from build123d import *

# Parameters (mm, degrees)
F0_R     = 5.0038
F0_R_2   = 5.1038
F0_R_3   = 5.2038
F0_R_4   = 5.3038
F0_R_5   = 5.4038
F0_R_6   = 5.9038
F0_R_7   = 5.8038
F0_R_8   = 5.7038
F0_R_9   = 5.6038
F0_R_10  = 5.5038
F1_DEPTH = 2.9464
F2_R     = 5.9038
F2_R_2   = 5.8038
F2_R_3   = 5.7038
F2_R_4   = 5.6038
F2_R_5   = 5.5038
F2_R_6   = 5.0038
F2_R_7   = 5.1038
F2_R_8   = 5.2038
F2_R_9   = 5.3038
F2_R_10  = 5.4038
F3_DEPTH = 2.54


with BuildPart() as f1:
    # F0 (on Top) → F1 (new body)
    with BuildSketch(Plane.XY):
        with BuildLine():
            Line((27.8450359044, 20.32), (-38.1949640956, 20.32))
            Line((-38.1949640956, 20.32), (-38.1949640956, -1.27))
            ThreePointArc((-38.1949640956, -1.27), (-36.3350921561, -5.7601280605), (-31.8449640956, -7.62))
            Line((-31.8449640956, -7.62), (27.8450359044, -7.62))
            Line((27.8450359044, -7.62), (27.8450359044, 20.32))
        make_face()
        with Locations((-30.5749640956, 0)):
            Circle(F0_R, mode=Mode.SUBTRACT)
        with Locations((-17.8749640956, 0)):
            Circle(F0_R_2, mode=Mode.SUBTRACT)
        with Locations((-5.1749640956, 0)):
            Circle(F0_R_3, mode=Mode.SUBTRACT)
        with Locations((7.5250359044, 0)):
            Circle(F0_R_4, mode=Mode.SUBTRACT)
        with Locations((20.2250359044, 0)):
            Circle(F0_R_5, mode=Mode.SUBTRACT)
        with Locations((-30.5749640956, 12.7)):
            Circle(F0_R_6, mode=Mode.SUBTRACT)
        with Locations((-17.8749640956, 12.7)):
            Circle(F0_R_7, mode=Mode.SUBTRACT)
        with Locations((-5.1749640956, 12.7)):
            Circle(F0_R_8, mode=Mode.SUBTRACT)
        with Locations((7.5250359044, 12.7)):
            Circle(F0_R_9, mode=Mode.SUBTRACT)
        with Locations((20.2250359044, 12.7)):
            Circle(F0_R_10, mode=Mode.SUBTRACT)
    extrude(amount=F1_DEPTH)

    # F2 (on face) → F3 (join)
    with BuildSketch(Plane(origin=(0, 0, 0), x_dir=(1, 0, 0), z_dir=(0, 0, -1))):
        with BuildLine():
            Line((-38.1949640956, 1.27), (-38.1949640956, -20.32))
            Line((-38.1949640956, -20.32), (27.8450359044, -20.32))
            Line((27.8450359044, -20.32), (27.8450359044, 7.62))
            Line((27.8450359044, 7.62), (-31.8449640956, 7.62))
            ThreePointArc((-31.8449640956, 7.62), (-36.3350921561, 5.7601280605), (-38.1949640956, 1.27))
        make_face()
        with Locations((-30.5749640956, -12.7)):
            Circle(F2_R, mode=Mode.SUBTRACT)
        with Locations((-17.8749640956, -12.7)):
            Circle(F2_R_2, mode=Mode.SUBTRACT)
        with Locations((-5.1749640956, -12.7)):
            Circle(F2_R_3, mode=Mode.SUBTRACT)
        with Locations((7.5250359044, -12.7)):
            Circle(F2_R_4, mode=Mode.SUBTRACT)
        with Locations((20.2250359044, -12.7)):
            Circle(F2_R_5, mode=Mode.SUBTRACT)
        with Locations((-30.5749640956, 0)):
            Circle(F2_R_6, mode=Mode.SUBTRACT)
        with Locations((-17.8749640956, 0)):
            Circle(F2_R_7, mode=Mode.SUBTRACT)
        with Locations((-5.1749640956, 0)):
            Circle(F2_R_8, mode=Mode.SUBTRACT)
        with Locations((7.5250359044, 0)):
            Circle(F2_R_9, mode=Mode.SUBTRACT)
        with Locations((20.2250359044, 0)):
            Circle(F2_R_10, mode=Mode.SUBTRACT)
        with Locations((-30.5749640956, 0)):
            Circle(F2_R_6)
        with Locations((-30.5749640956, -12.7)):
            Circle(F2_R)
        with Locations((-17.8749640956, -12.7)):
            Circle(F2_R_2)
        with Locations((-17.8749640956, 0)):
            Circle(F2_R_7)
        with Locations((-5.1749640956, 0)):
            Circle(F2_R_8)
        with Locations((-5.1749640956, -12.7)):
            Circle(F2_R_3)
        with Locations((7.5250359044, -12.7)):
            Circle(F2_R_4)
        with Locations((7.5250359044, 0)):
            Circle(F2_R_9)
        with Locations((20.2250359044, 0)):
            Circle(F2_R_10)
        with Locations((20.2250359044, -12.7)):
            Circle(F2_R_5)
    extrude(amount=F3_DEPTH)


solid = f1.part
The listing builds one solid part. Answer for the finished solid, in the listing's coordinates (mm). A direction names the side the tool comes from. Coordinates: 2 decimals unless noted, no trailing zeros. Loops run counter-clockwise (first coordinate to the right, second up) from the corner with the lowest first, then second, coordinate; pieces in that order, holes last. Notation, with made-up numbers: (89, -0.5) -> (121, -0.5) arc R33 cw to (121, 31.5) -> close; hole circle Ø6 at (81, 6.5). An arc over 180 degrees is marked (long way). Answer in a Markdown table with one row per item. Add a question column.
1. For faces 1 (the flat face through (-38.195, 9, 0)), 2 (the flat face through (-5, 0, 0)), determine the directions among +Z, -Z, +X, -X, +Y, -Y from which every point of the face is accessible in a straight line to the end or side of a thin tool.
2. Determine the mould class of faces 3 (the cylindrical face through (-36.285, -5.809, 0.242)), 4 (the flat face through (27.845, 7, 0)), 5 (the cylindrical face through (14.826, 0.238, 1.453)), 6 (the flat face through (-6, 20.32, 0)) for opening direction X: +X half, -X half, draft (parallel to the pull), parting line (faces both ways), or undercut.
3. The part is cut by section D-D, the plane y = 0. Write down the section's boundary in (x, z).
4. The part is cut by section C-C, the plane x = -31. Write down the section's boundary in (y, z), then the cut area to 3 significant figures.
5. Flat-ended cylindrical pins translate along their axes: P1, Ø13, axis at x = -30.5, y = 14.5, coming from the +Z side; P2, Ø10.5, axis at x = -30.57, y = 12.7, coming from the +Z side. Find the tip coordinate at first contact, or state that the pin passes through.
6. Consider line 1 (X direction, y = -4, z = 0.15); line 2 (X direction, y = 3, z = 1.35); line 3 (Z direction, x = 17, y = 1). Determine where each line is inside the solid, lowest interval first. Write a range as [from, to].
7. The part is cut by section A-A, the plane z = 0.75. Count the separate pieces of the cut face and the enclosed holes in it, then the cut area to 3 significant figures.
8. The part is cut by section B-B, the plane y = 12.7. Write down the section's boundary in (x, z), then the cut area to 3 significant figures.
Answer below:
| question | item | result |
|---|---|---|
| 1 | face 1 | +Z, -Z, -X, +Y, -Y |
| 1 | face 2 | +Z |
| 2 | face 3 | -X half |
| 2 | face 4 | +X half |
| 2 | face 5 | undercut |
| 2 | face 6 | draft |
| 3 | outline | (-38.19, -2.54) -> (27.85, -2.54) -> (27.85, 2.95) -> (25.63, 2.95) -> (25.63, 0) -> (14.82, 0) -> (14.82, 2.95) -> (12.83, 2.95) -> (12.83, 0) -> (2.22, 0) -> (2.22, 2.95) -> (0.03, 2.95) -> (0.03, 0) -> (-10.38, 0) -> (-10.38, 2.95) -> (-12.77, 2.95) -> (-12.77, 0) -> (-22.98, 0) -> (-22.98, 2.95) -> (-25.57, 2.95) -> (-25.57, 0) -> (-35.58, 0) -> (-35.58, 2.95) -> (-38.19, 2.95) -> close |
| 4 | outline | (-7.62, -2.54) -> (20.32, -2.54) -> (20.32, 2.95) -> (18.59, 2.95) -> (18.59, 0) -> (6.81, 0) -> (6.81, 2.95) -> (4.99, 2.95) -> (4.99, 0) -> (-4.99, 0) -> (-4.99, 2.95) -> (-7.62, 2.95) -> close |
| 4 | area | 89.2 mm2 |
| 5 | P1 | z = 2.95 |
| 5 | P2 | z = 0 |
| 6 | line 1 | [-37.58, -33.58], [-27.57, -21.04], [-14.7, -8.5], [-1.85, 4.04], [11.01, 16.59], [23.86, 27.85] |
| 6 | line 2 | [-38.19, -34.58], [-26.57, -22], [-13.75, -9.43], [-0.92, 3.15], [11.9, 15.73], [24.72, 27.85] |
| 6 | line 3 | [-2.54, 0] |
| 7 | separate pieces | 1 |
| 7 | enclosed holes | 10 |
| 7 | area | 899 mm2 |
| 8 | outline | (-38.19, -2.54) -> (27.85, -2.54) -> (27.85, 2.95) -> (25.73, 2.95) -> (25.73, 0) -> (14.72, 0) -> (14.72, 2.95) -> (13.13, 2.95) -> (13.13, 0) -> (1.92, 0) -> (1.92, 2.95) -> (0.53, 2.95) -> (0.53, 0) -> (-10.88, 0) -> (-10.88, 2.95) -> (-12.07, 2.95) -> (-12.07, 0) -> (-23.68, 0) -> (-23.68, 2.95) -> (-24.67, 2.95) -> (-24.67, 0) -> (-36.48, 0) -> (-36.48, 2.95) -> (-38.19, 2.95) -> close |
| 8 | area | 194 mm2 |
